The listing builds one solid part. Answer for the finished solid, in the listing's coordinates (mm). Face numbers are marked on the shaded views. A direction names the side the tool comes from. Coordinates: 2 decimals unless noted, no trailing zeros. Write each loop counter-clockwise with the first axis right and the second up, starting at its lowest first coordinate (ties: lowest second). Pieces come first, ordered by that corner, then holes.
(1) The part is cut by section D-D on y = 10.5. Determine the outline of the cut face in (x, z) (3 decimals), plus the area to 3 significant figures.
(2) The part is cut by section B-B on z = -5.5. Determine the outline of the cut face in (x, y) (3 decimals), plus the area to 3 significant figures.
(3) Given P1, Ø1.5, axis at x = -16.5, z = -4, coming from the +Y side (3 decimals); P2, Ø10, axis at x = -11.5, y = 13, coming from the -Z side; P3, Ø8, axis at y = 13, z = -14.5, coming from the +X side, each flat-ended and moving along its own axis, determine where each tip first touches the part or whether it passes through.
(4) Straight lines are drawn through the part: line 1 (X direction, y = 2.5, z = -12.7) (3 decimals); line 2 (Y direction, x = -10.25, z = -11) (3 decimals); line 3 (X direction, y = 3.75, z = -16.75) (3 decimals). For each, find the intervals that lie inside material, in ascending order.
(5) The part is cut by section A-A on x = -12.7. Determine the outline of the cut face in (y, z) (3 decimals), plus the area to 3 significant figures.
(6) Which of the six approach directions +Z, -Z, +X, -X, +Y, -Y give full straight-line access (tool end or side, diameter ignored) to the marked faces 1 and 2?
(7) The part is cut by section C-C on z = -12.7. Determine the outline of the cut face in (x, y) (3 decimals).
Autodesk Inventor part; units mm, degrees
ref_plane "YZ Plane" through (0, 0, 0) normal (1, 0, 0) x (0, 1, 0)
ref_plane "XZ Plane" through (0, 0, 0) normal (0, 1, 0) x (-1, 0, 0)
ref_plane "XY Plane" through (0, 0, 0) normal (0, 0, 1) x (1, 0, 0)
sketch "Sketch1" plane through (0, 0, 0) normal (0, 1, 0) x (-1, 0, 0)
  line L0 (0, 0) -> (25.4, 0)
  line L1 (25.4, 0) -> (25.4, -25.4)
  line L2 (25.4, -25.4) -> (0, -25.4)
  line L3 (0, -25.4) -> (0, 0)
  dimension "d0" = 25.4
  dimension "d1" = 25.4
extrude "Extrusion1" add sketch "Sketch1" along normal blind 3.175
sketch "Sketch2" plane through (0, 0, 0) normal (0, 1, 0) x (1, 0, 0)
  line L0 (-25.4, 0) -> (0, 0) construction
  line L1 (-12.7, 0) -> (-12.7, 12.7) construction
  line L2 (0, 25.4) -> (-25.4, 25.4) construction
  line L3 (-12.7, 25.4) -> (-12.7, 12.7) construction
  line L4 (-25.4, 25.4) -> (-25.4, 0) construction
  line L5 (-25.4, 12.7) -> (0, 12.7) construction
  line L6 (-25.4, 25.4) -> (-28.575, 25.4)
  line L7 (-28.575, 25.4) -> (-28.575, 0)
  line L8 (-28.575, 0) -> (-25.4, 0)
  line L9 (-25.4, 0) -> (-25.4, 25.4)
  dimension "d4" = 12.7
  dimension "d5" = 12.7
  dimension "d6" = 3.175
extrude "Extrusion2" add sketch "Sketch2" along normal blind 28.575
sketch "Sketch3" plane through (0, 3.175, 0) normal (0, 1, 0) x (1, 0, 0)
  line L0 (0, 0) -> (0, 25.4) construction
  line L1 (0, 12.7) -> (-16.1864, 12.7) construction
  line L2 (0, 25.4) -> (-25.4, 25.4) construction
  line L3 (-12.7, 25.4) -> (-12.7, 5.173) construction
  circle A0 centre (-12.7, 12.7) radius 2.5797
  dimension "d9" = 5.1594
sketch "Sketch4" plane through (-25.4, 3.175, -25.4) normal (1, 0, 0) x (0, 0, -1)
  line L0 (0, 25.4) -> (-25.4, 25.4) construction
  line L1 (-12.7, 25.4) -> (-12.7, 8.5615) construction
  line L2 (-25.4, -3.175) -> (-25.4, 25.4) construction
  line L3 (-25.4, 11.1125) -> (0.5761, 11.1125) construction
  circle A0 centre (-12.412, 11.1125) radius 2.5797
  dimension "d10" = 5.1594
extrude "Extrusion3" cut sketch "Sketch4" against normal blind 28.575
extrude "Extrusion4" cut sketch "Sketch3" against normal blind 28.575
properties part number "spring extentsion"
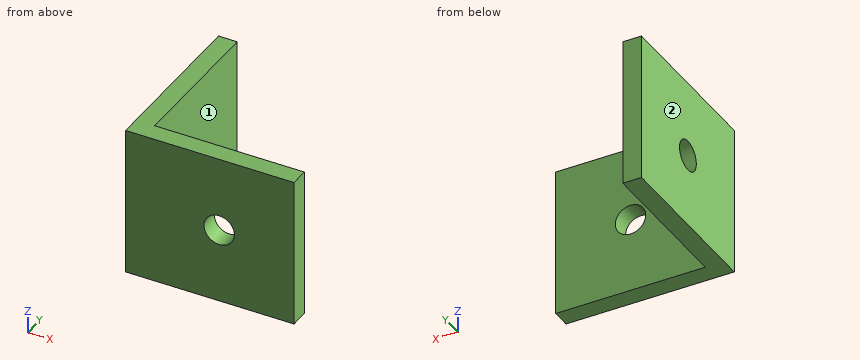
Model answer:
1. outline: (-28.575, -25.4) - (-25.4, -25.4) - (-25.4, 0) - (-28.575, 0) - close
1. area: 80.6 mm2
2. outline: (-28.575, 0) - (0, 0) - (0, 3.175) - (-25.4, 3.175) - (-25.4, 28.575) - (-28.575, 28.575) - close
2. area: 171 mm2
3. P1: stops at y = 3.175
3. P2: passes through
3. P3: stops at x = -25.4
4. line 1: x = -28.575 to -15.28, -10.12 to 0
4. line 2: y = 0 to 3.175
4. line 3: x = -28.575 to -25.4
5. outline: (0, -25.4) - (3.175, -25.4) - (3.175, -15.28) - (0, -15.28) - close; (0, -10.12) - (3.175, -10.12) - (3.175, 0) - (0, 0) - close
5. area: 64.3 mm2
6. face 1: +Z, -Z, +X, +Y
6. face 2: +Z, -Z, -X, +Y, -Y
7. outline: (-28.575, 0) - (-15.28, 0) - (-15.28, 3.175) - (-25.4, 3.175) - (-25.4, 11.724) - (-28.575, 11.724) - close; (-28.575, 16.851) - (-25.4, 16.851) - (-25.4, 28.575) - (-28.575, 28.575) - close; (-10.12, 0) - (0, 0) - (0, 3.175) - (-10.12, 3.175) - close
